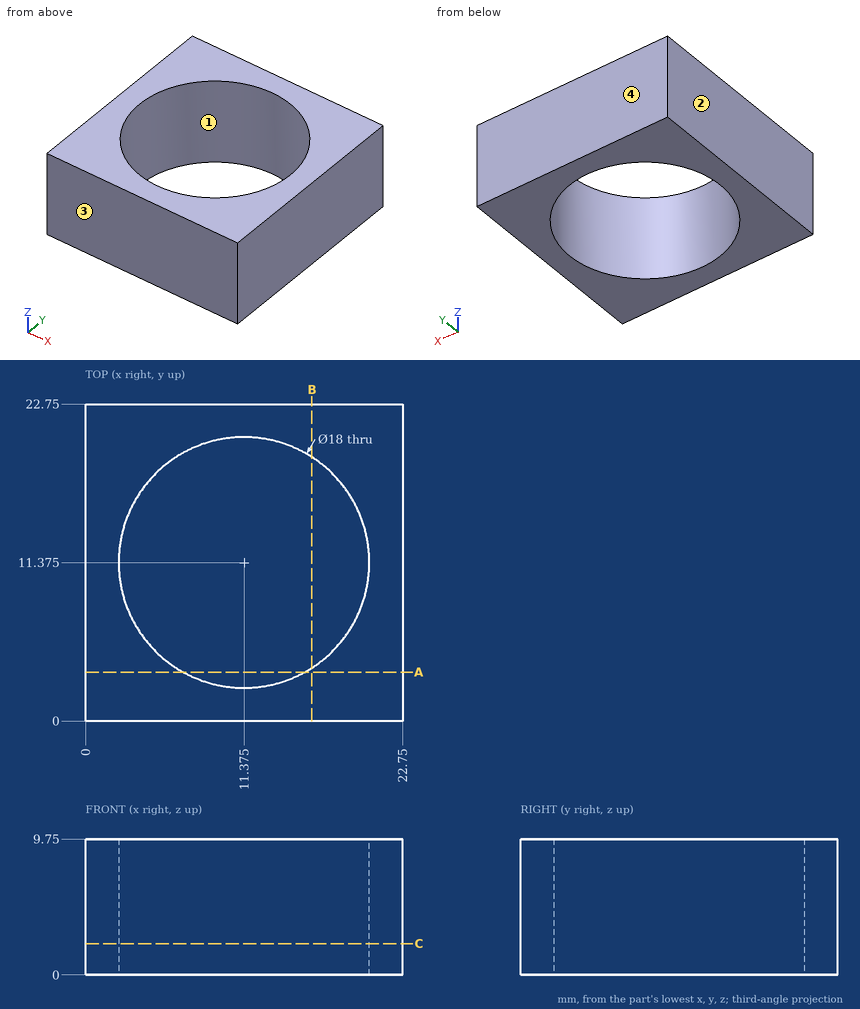
Answer from the drawing. Dimensions are ordinates in mm from the lowest x, y and z of the part. Coordinates: 2 decimals unless noted, no trailing zeros. Order: outer loops, then holes, each group sorted by start corner. A loop starts at its lowest first (then second) coordinate and runs counter-clockwise, first axis right, second up. Notation, with made-up numbers: (-25.5, 89.25) -> (-7.5, 89.25) arc R26 ccw to (-7.5, 126.25) -> close; hole circle Ø1 at (-14.75, 3). An arc over 180 degrees is marked (long way). Answer as a JSON object with one key per item and string values.
1) A cutting plane is placed at A-A, the plane y = 3.5. Determine the outline of the cut face in (x, z), plus the area to 3 significant figures.
Model answer:
{"outline": "(0, 0) -> (7.02, 0) -> (7.02, 9.75) -> (0, 9.75) -> close; (15.73, 0) -> (22.75, 0) -> (22.75, 9.75) -> (15.73, 9.75) -> close", "area": "137 mm²"}
2) A cutting plane is placed at C-C, the plane z = 2.25. Determine the outline of the cut face in (x, y) (3 decimals), plus the area to 3 significant figures.
Model answer:
{"outline": "(0, 0) -> (22.75, 0) -> (22.75, 22.75) -> (0, 22.75) -> close; hole circle Ø18 at (11.375, 11.375)", "area": "263 mm²"}
3) Consider line 1 along X through (y, z) = (3.25, 9.25); line 2 along Y through (x, z) = (10.75, 7.5); line 3 along Y through (x, z) = (4, 4.25). Determine where each line is inside the solid, lowest interval first. Write a range as from..to.
Model answer:
{"line 1": "x = 0..7.5, 15.25..22.75", "line 2": "y = 0..2.4, 20.35..22.75", "line 3": "y = 0..6.22, 16.53..22.75"}
4) The mould has two halves that part along Y. Classify the marked faces 1, 2, 3 and 4: released by +Y, released by -Y, zero draft, split by the parting line, or undercut.
Model answer:
{"face 1": "undercut", "face 2": "zero draft", "face 3": "released by -Y", "face 4": "released by +Y"}
5) A cutting plane is placed at B-B, the plane x = 16.25. Determine the outline of the cut face in (y, z).
Model answer:
{"outline": "(0, 0) -> (3.81, 0) -> (3.81, 9.75) -> (0, 9.75) -> close; (18.94, 0) -> (22.75, 0) -> (22.75, 9.75) -> (18.94, 9.75) -> close"}
